Model file for the job. Use its own axes, mm. A direction names the side the tool comes from. Give positions to 0.01 mm unless a question says otherwise; leave off trailing zeros. Order: outer loops, then holes, each group sorted by start corner. A loop starts at its lowest first (then second) coordinate and runs counter-clockwise, first axis right, second up. Notation, with made-up numbers: M 9,23.25 L 58,23.25 A21 cw 58,48.25 Z; hole C -21,11.5 d3. An arc over 180 degrees is marked long. Return JSON: item names as keys, results as strings. Group by question number.
1. 3-axis set-ups, long thin cutter, end or side, ignore diameter. For faces 1 (the face through (-2.535, -4.31, 2.099)), 2 (the face through (-5, 0, 2)), 3 (the face through (-2.465, 4.35, 2.099)): which of +Z, -Z, +X, -X, +Y, -Y reach the whole face in a straight line?
2. Pin check, flat tips, straight feed: pin 1 (0.8 mm diameter, centred on y = 0, z = 1.5, fed in from +X); pin 2 (2 mm diameter, centred on x = 0.5, y = -1.5, fed in from -Z); pin 3 (2 mm diameter, centred on y = 0, z = 2.5, fed in from -X); pin 4 (3 mm diameter, centred on x = 0, y = 0, fed in from -Z). Stop position of each tip, or through.
3. Slice it at A-A on y = 0. List the corners of the cut face in (x, z).
4. Slice it at B-B on z = 1.7. List the corners of the cut face in (x, y).
5. Slice it at C-C on z = 3.7. List the corners of the cut face in (x, y).
6. Wall check: probe 1 along Z at (x, y) = (-3, 4.25); probe 2 along Y at (x, z) = (1, 2.8); probe 3 along X at (y, z) = (-1, 2.3). Give the ranges that are in metal, low to high. Write a range as [from, to].
7. Two-plate mould, pull along Y, no slides. Class faces 4 (the face through (2.535, 4.31, 2.099)), 5 (the face through (0.54, -2.44, 1.98)), 6 (the face through (2.6, 4.5, 0.8)), 7 (the face through (2.465, -4.35, 2.099)): released by +Y, released by -Y, zero draft, split by the parting line, or undercut.
from build123d import *

# Parameters (mm, degrees)
SKETCH_1_R          = 6
EXTRUDE_1_DEPTH     = 0.8
EXTRUDE_2_DEPTH     = 3.2
SKETCH_3_OUTSIDE_W  = 38.42
SKETCH_3_OUTSIDE_H  = 38.42
SKETCH_3_OUTSIDE_R  = 3.15
CUT_EXTRUDE_1_DEPTH = 3.2
CUT_EXTRUDE_1_DRAFT = -73
HOLE_WIZARD_M61_D   = 5
CHAMFER_1_SIZE      = 0.5
CHAMFER_2_SIZE      = 0.5


with BuildPart() as part:
    # Эскиз1 → Бобышка-Вытянуть1 (new body)
    with BuildSketch(Plane.XY):
        Circle(SKETCH_1_R)
    extrude(amount=EXTRUDE_1_DEPTH)

    # Эскиз2 → Бобышка-Вытянуть2 (add)
    with BuildSketch(Plane.XY.offset(0.8)):
        Polygon((0, 5.773502692), (-5, 2.886751346), (-5, -2.886751346), (0, -5.773502692), (5, -2.886751346), (5, 2.886751346), align=None)
    extrude(amount=EXTRUDE_2_DEPTH)


with BuildPart() as cut_extrude_1_tool:
    # Эскиз3 outside → Вырез-Вытянуть1 (with draft: the straight prism first)
    with BuildSketch(Plane.XY.offset(4)):
        Rectangle(SKETCH_3_OUTSIDE_W, SKETCH_3_OUTSIDE_H)
        Circle(SKETCH_3_OUTSIDE_R, mode=Mode.SUBTRACT)
    extrude(amount=-CUT_EXTRUDE_1_DEPTH)
    # Вырез-Вытянуть1: the draft: its side faces are tilted about the plane it starts from
    cut_extrude_1_sides = [cut_extrude_1_tool.faces().sort_by_distance(p)[0] for p in [
        (0, -19.21, 2.4),
        (19.21, 0, 2.4),
        (0, 19.21, 2.4),
        (-19.21, 0, 2.4),
        (-3.15, 0, 2.4),
    ]]
    draft(cut_extrude_1_sides, Plane.XY.offset(4), CUT_EXTRUDE_1_DRAFT)


with BuildPart() as part_1:
    add(part.part)

    # Вырез-Вытянуть1: cut by cut_extrude_1_tool
    add(cut_extrude_1_tool.part, mode=Mode.SUBTRACT)

    # Отверстие обработанное метчиком M61 (through all)
    with Locations(Plane.XY.offset(4)):
        with Locations((0, 0)):
            Hole(HOLE_WIZARD_M61_D / 2)

    # Фаска1
    chamfer_1_edges = [part_1.edges().sort_by_distance(p)[0] for p in [
        (2.5, 0, 4),
    ]]
    chamfer(chamfer_1_edges, length=CHAMFER_1_SIZE)

    # Фаска2
    chamfer_2_edges = [part_1.edges().sort_by_distance(p)[0] for p in [
        (2.5, 0, 0),
    ]]
    chamfer(chamfer_2_edges, length=CHAMFER_2_SIZE)


solid = part_1.part
Result:
{
 "1": {"face 1": "+Z, -X, -Y", "face 2": "+Z, -X, +Y, -Y", "face 3": "+Z, -X, +Y"},
 "2": {"pin 1": "stops at x = 5", "pin 2": "stops at z = 0.42", "pin 3": "stops at x = -5", "pin 4": "passes through"},
 "3": {"outline": "M -6,0 L -3,0 L -2.5,0.5 L -2.5,3.5 L -3,4 L -3.15,4 L -5,3.43 L -5,0.8 L -6,0.8 Z; M 2.5,0.5 L 3,0 L 6,0 L 6,0.8 L 5,0.8 L 5,3.43 L 3.15,4 L 3,4 L 2.5,3.5 Z"},
 "4": {"outline": "M -5,-2.89 L 0,-5.77 L 5,-2.89 L 5,2.89 L 0,5.77 L -5,2.89 Z; hole C 0,0 d5"},
 "5": {"outline": "C 0,0 d8.26; hole C 0,0 d5.4"},
 "6": {"probe 1": "z = [0, 0.8]", "probe 2": "y = [-5.2, -2.29], [2.29, 5.2]", "probe 3": "x = [-5, -2.29], [2.29, 5]"},
 "7": {"face 4": "released by +Y", "face 5": "undercut", "face 6": "zero draft", "face 7": "released by -Y"}
}
